The figure shows three views and two pictorial views of one solid part (mm, origin at its lowest corner). Answer the questions. Coordinates: 2 decimals unless noted, no trailing zeros. Write each loop counter-clockwise with the first axis right and the second up, starting at its lowest first coordinate (ties: lowest second). Pieces come first, ordered by that corner, then holes. Notation, with made-up numbers: (78.25, -21.5) - (85.25, -21.5) arc R10 cw to (85.25, -7.5) - close; hole circle Ø9 at (43, 60). An arc over 180 degrees is marked (long way). Use a Markdown table: item, result. Add a question column.
(1) The part is cut by section B-B, the plane z = 12.75. Give the vertices of the cut face in (x, y) (1 decimal).
(2) Given pin 1 Ø4 at (x, y) = (4.97, 5.02) entering from -Z, flat-ended and moving along its own axis, determine where the tip first touches the part or whether it passes through.
(3) For a pull along Y with two mould halves and no side action, classify the marked faces 1, 2, 3 and 4 as released by +Y, released by -Y, zero draft, split by the parting line, or undercut.
(4) Find the intervals of material crossed by line 1 (Y direction, x = 5, z = 1.5); line 2 (X direction, y = 3.25, z = 3.75); line 3 (Y direction, x = 6.25, z = 5.25) (1 decimal), in increasing order. Write a range as from..to.
(5) The part is cut by section A-A, the plane y = 1.5. Give the vertices of the cut face in (x, z), then the cut area to 3 significant figures.
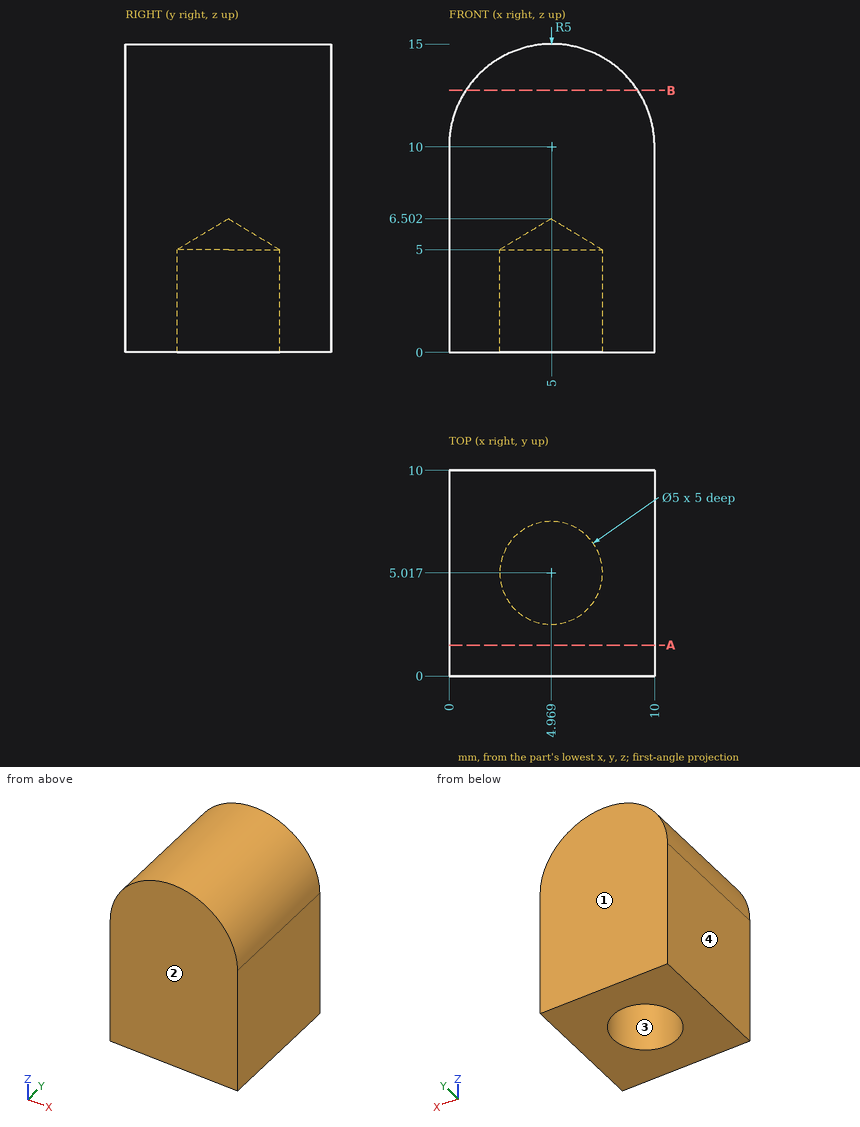
Model answer:
| question | item | result |
|---|---|---|
| 1 | outline | (0.8, 0) - (9.2, 0) - (9.2, 10) - (0.8, 10) - close |
| 2 | pin 1 | z = 5.3 |
| 3 | face 1 | released by +Y |
| 3 | face 2 | released by -Y |
| 3 | face 3 | undercut |
| 3 | face 4 | zero draft |
| 4 | line 1 | 0..2.52, 7.52..10 |
| 4 | line 2 | 0..3.2, 6.74..10 |
| 4 | line 3 | 0..3.4, 6.7..10 |
| 5 | outline | (0, 0) - (10, 0) - (10, 10) arc R5 ccw to (0, 10) - close |
| 5 | area | 139 mm^2 |
